Build history of the part. All positions in model axes, mm. A direction names the side the tool comes from. Coordinates: 2 decimals unless noted, no trailing zeros. Order: outer loops, then holes, each group sorted by start corner. A loop starts at its lowest first (then second) coordinate and runs counter-clockwise, first axis right, second up. Notation, with made-up numbers: (63, -10) -> (116, -10) arc R24 ccw to (116, 7) -> close; hole circle Ø4 at (52.5, 47). An arc over 180 degrees is marked (long way). Write each question's results on one line, items separated by ' | '.
from build123d import *

# Parameters (mm, degrees)
SKETCH4_R          = 30
CUT_EXTRUDE3_DEPTH = 1
SKETCH5_R          = 2
CUT_EXTRUDE4_DEPTH = 6


with BuildPart() as part:
    # Sketch2 → Revolve-Thin1 (revolve)
    with BuildSketch(Plane.XY, mode=Mode.PRIVATE) as revolve_thin1_sk:
        Polygon((-30.230643129, 25.839523207), (-6.494921795, 25.839523207), (-6.494921795, 21.839523207), (-6.494921795, 0.092953851), (1.505078205, 0.092953851), (1.505078205, -3.652740104), (-2.730643129, -20.632394541), (-2.730643129, -23.886700586), (-5.730643129, -23.886700586), (-5.730643129, -30.625568886), (-5.730643129, -38.610085728), (-17.730643129, -38.610085728), (-17.730643129, 12.839523207), (-30.230643129, 12.839523207), align=None)
        Polygon((-28.230643129, 23.839523207), (-8.494921795, 23.839523207), (-8.494921795, 21.839523207), (-8.494921795, -1.907046149), (-0.494921795, -1.907046149), (-0.494921795, -3.407046149), (-4.730643129, -20.386700586), (-4.730643129, -21.886700586), (-7.730643129, -21.886700586), (-7.730643129, -30.625568886), (-7.730643129, -36.610085728), (-15.730643129, -36.610085728), (-15.730643129, 14.839523207), (-28.230643129, 14.839523207), align=None, mode=Mode.SUBTRACT)
    revolve(revolve_thin1_sk.sketch.rotate(Axis((14.769356871, -26.256134736, 0), (0, 1, 0)), 270), axis=Axis((14.769356871, -26.256134736, 0), (0, 1, 0)))

    # Sketch4 → Cut-Extrude3 (cut)
    with BuildSketch(Plane(origin=(0, 25.839523207, 0), x_dir=(1, 0, 0), z_dir=(0, 1, 0))):
        with Locations(Location((14.769356871, 0, 0), (0, 0, 270))):
            Circle(SKETCH4_R)
    extrude(amount=-CUT_EXTRUDE3_DEPTH, mode=Mode.SUBTRACT)

    # Sketch5 → Cut-Extrude4 (cut)
    with BuildSketch(Plane(origin=(0, 25.839523207, 0), x_dir=(1, 0, 0), z_dir=(0, 1, 0))):
        with Locations(Location((14.769356871, 26, 0), (0, 0, 270))):
            Circle(SKETCH5_R)
        with Locations(Location((37.28601737, 13, 0), (0, 0, 270))):
            Circle(SKETCH5_R)
        with Locations(Location((37.28601737, -13, 0), (0, 0, 270))):
            Circle(SKETCH5_R)
        with Locations(Location((14.769356871, -26, 0), (0, 0, 270))):
            Circle(SKETCH5_R)
        with Locations(Location((-7.747303627, -13, 0), (0, 0, 270))):
            Circle(SKETCH5_R)
        with Locations(Location((-7.747303627, 13, 0), (0, 0, 270))):
            Circle(SKETCH5_R)
    extrude(amount=-CUT_EXTRUDE4_DEPTH, mode=Mode.SUBTRACT)


solid = part.part
Item 1: Pin check, flat tips, straight feed: pin 1 (6.5 mm diameter, centred on x = 37.29, z = -13, fed in from +Y); pin 2 (5 mm diameter, centred on x = 10.5, y = 18.5, fed in from +Z); pin 3 (24 mm diameter, centred on x = 14.77, z = 0, fed in from -Y); pin 4 (3 mm diameter, centred on x = -1, y = -18.5, fed in from +Z). Stop position of each tip, or through.
Answer:
pin 1: stops at y = 24.84 | pin 2: stops at z = 44.97 | pin 3: passes through | pin 4: stops at z = 29.2
Item 2: Slice it at B-B, the plane x = 40.5. List the corners of the cut face in (y, z), and give its area (3 significant figures).
Answer:
outline: (-38.61, -19.85) -> (12.84, -19.85) -> (12.84, -36.92) -> (25.84, -36.92) -> (25.84, -15.43) -> (24.84, -15.43) -> (24.84, 15.43) -> (25.84, 15.43) -> (25.84, 36.92) -> (12.84, 36.92) -> (12.84, 19.85) -> (-38.61, 19.85) -> close; hole (-36.61, -16.38) -> (14.84, -16.38) -> (14.84, -34.45) -> (23.84, -34.45) -> (23.84, 34.45) -> (14.84, 34.45) -> (14.84, 16.38) -> (-36.61, 16.38) -> close | area: 667 mm^2
Item 3: Tool access for faces 1 (the flat face through (14, -38.61, 21)), 2 (the cylindrical face through (27.22, -12.53, -30.02)), 3 (the flat face through (-4, -21.887, -7)), 4 (the cylindrical face through (-14.52, 25.35, -6.5)), 5 (the cylindrical face through (1.62, -1.81, 1.73)): list every direction of +Z, -Z, +X, -X, +Y, -Y with a clear straight run to the whole face (end or side of a thin tool).
Answer:
face 1: +Z, -Z, +X, -X, -Y | face 2: -Y | face 3: none | face 4: +Y | face 5: +Y, -Y
Item 4: Slice it at A-A, the plane z = 0. State how many separate pieces and enclosed holes the cut face has, and give its area (3 significant figures).
Answer:
separate pieces: 2 | enclosed holes: 2 | area: 705 mm^2
Item 5: Slice it at D-D, the plane z = -37.5. List the corners of the cut face in (x, y), and give its area (3 significant figures).
Answer:
outline: (-10.11, 12.84) -> (39.64, 12.84) -> (39.64, 25.84) -> (-10.11, 25.84) -> close; hole (-6.27, 14.84) -> (35.81, 14.84) -> (35.81, 23.84) -> (-6.27, 23.84) -> close | area: 268 mm^2
Item 6: Pull direction Y, two halves, no side cores. Call faces 6 (the cylindrical face through (-9.7, 24.35, -13.43)), 7 (the cylindrical face through (36.734, -29.351, 4.878)), 8 (the flat face through (45, 12.84, 13)): released by +Y, released by -Y, zero draft, split by the parting line, or undercut.
Answer:
face 6: zero draft | face 7: undercut | face 8: released by -Y
Item 7: Slice it at C-C, the plane y = 8. List the corners of the cut face in (x, z), and give its area (3 significant figures).
Answer:
outline: circle Ø65 at (14.77, 0); circle Ø46.53 at (14.77, 0); hole circle Ø61 at (14.77, 0); hole circle Ø42.53 at (14.77, 0) | area: 676 mm^2
Item 8: Drill centre lines: line 1 (X direction, y = -2.5, z = 0); line 2 (X direction, y = -1.8, z = 0); line 3 (Y direction, x = 8, z = -40). Where is each one in solid material? Low to high. Write a range as from..to.
Answer:
line 1: x = -17.73..-15.73, -0.49..1.51, 28.03..30.03, 45.27..47.27 | line 2: x = -17.73..-15.73, -8.49..1.51, 28.03..38.03, 45.27..47.27 | line 3: y = 12.84..14.84, 23.84..25.84
